Verification items for the finished model (mm, model axes). Face numbers are marked on the shaded views. A direction names the side the tool comes from. Give positions to 0.01 mm unless a question says otherwise; leave off trailing zeros. Loops run counter-clockwise (first coordinate to the right, second up) from the corner with the lowest first, then second, coordinate; pieces in that order, holes last. Notation, with made-up numbers: (36.5, 42.25) - (79.5, 42.25) arc R17 cw to (79.5, 69.25) - close; hole circle Ø6 at (80.25, 73). An arc over 180 degrees is marked (long way). Use one line per item in the form item = value.
```python
from build123d import *

# Parameters (mm, degrees)
F0_R      = 6.6
F1_DEPTH  = 7
F2_R      = 6.55
F3_DEPTH  = 7
F4_R      = 6.5
F5_DEPTH  = 7
F6_R      = 6.45
F7_DEPTH  = 7
F8_R      = 6.4
F9_DEPTH  = 7
F10_R     = 6.35
F11_DEPTH = 7
F12_R     = 6.3
F13_DEPTH = 7
F14_R     = 6.25
F15_DEPTH = 7
F16_R     = 6.2
F17_DEPTH = 7
F18_R     = 6.15
F19_DEPTH = 7
F20_R     = 6.1
F21_DEPTH = 7
F22_R     = 6.05
F23_DEPTH = 7
F24_R     = 6
F25_DEPTH = 7


# Not quite as in the source:
# - a feature of the source that left no trace in its solid (it failed there, or was rolled back) is left out


with BuildPart() as f1:
    # F0 (on Top) → F1 (new body)
    with BuildSketch(Plane.XY):
        Circle(F0_R)
    extrude(amount=F1_DEPTH)

    # F2 (on face) → F3 (join)
    with BuildSketch(Plane.XY.offset(7)):
        Circle(F2_R)
    extrude(amount=F3_DEPTH)

    # F4 (on face) → F5 (join)
    with BuildSketch(Plane.XY.offset(14)):
        Circle(F4_R)
    extrude(amount=F5_DEPTH)

    # F6 (on face) → F7 (join)
    with BuildSketch(Plane.XY.offset(21)):
        Circle(F6_R)
    extrude(amount=F7_DEPTH)

    # F8 (on face) → F9 (join)
    with BuildSketch(Plane.XY.offset(28)):
        Circle(F8_R)
    extrude(amount=F9_DEPTH)

    # F10 (on face) → F11 (join)
    with BuildSketch(Plane.XY.offset(35)):
        Circle(F10_R)
    extrude(amount=F11_DEPTH)

    # F12 (on face) → F13 (join)
    with BuildSketch(Plane.XY.offset(42)):
        Circle(F12_R)
    extrude(amount=F13_DEPTH)

    # F14 (on face) → F15 (join)
    with BuildSketch(Plane.XY.offset(49)):
        Circle(F14_R)
    extrude(amount=F15_DEPTH)

    # F16 (on face) → F17 (join)
    with BuildSketch(Plane.XY.offset(56)):
        Circle(F16_R)
    extrude(amount=F17_DEPTH)

    # F18 (on face) → F19 (join)
    with BuildSketch(Plane.XY.offset(63)):
        Circle(F18_R)
    extrude(amount=F19_DEPTH)

    # F20 (on face) → F21 (join)
    with BuildSketch(Plane.XY.offset(70)):
        Circle(F20_R)
    extrude(amount=F21_DEPTH)

    # F22 (on face) → F23 (join)
    with BuildSketch(Plane.XY.offset(77)):
        Circle(F22_R)
    extrude(amount=F23_DEPTH)

    # F24 (on face) → F25 (join)
    with BuildSketch(Plane.XY.offset(84)):
        Circle(F24_R)
    extrude(amount=F25_DEPTH)


solid = f1.part
```
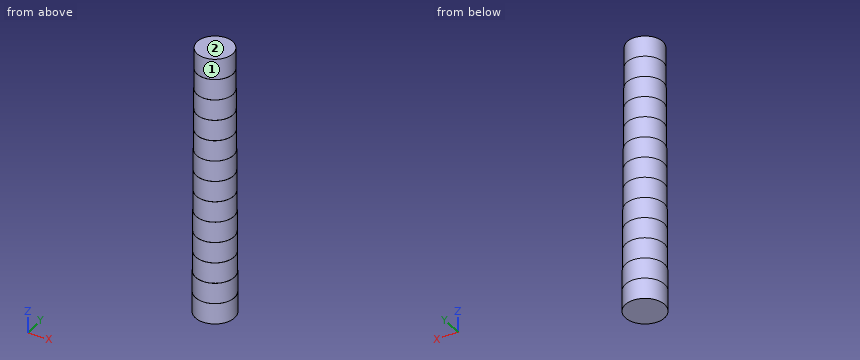
1. Depth check by flat-ended pin: pin 1 Ø1.5 at (y, z) = (-0.5, 58) entering from +X; pin 2 Ø5 at (x, z) = (0, 28.5) entering from +Y; pin 3 Ø6 at (x, z) = (-2, 53) entering from -Y. Enter the tip coordinate at first touch or a pass-through.
Result set:
pin_1 = 6.2
pin_2 = 6.45
pin_3 = -6.25
2. Tool access check on the marked faces 1 and 2. Record the directions out of +Z, -Z, +X, -X, +Y, -Y that give a thin tool (end or side, any length) a straight path to the whole face; none if there is none.
Result set:
face_1 = +Z
face_2 = +Z, +X, -X, +Y, -Y
3. Section check A-A, the plane z = 33. Record the cut outline in (x, y), then the cut area to 3 significant figures.
Result set:
outline = circle Ø12.8 at (0, 0)
area = 129 mm²
4. Scan lines: probe 1 along Y at (x, z) = (-1.75, 27.5); probe 2 along Y at (x, z) = (1, 65); probe 3 along X at (y, z) = (-5.25, 47). Record each from-to range of solid material in increasing order.
Result set:
probe_1 = -6.21 to 6.21
probe_2 = -6.07 to 6.07
probe_3 = -3.48 to 3.48
5. Section check B-B, the plane z = 15. Record the cut outline in (x, y), then the cut area to 3 significant figures.
Result set:
outline = circle Ø13 at (0, 0)
area = 133 mm²
